The drawing under review shows one solid part. Ordinate dimensions are in mm from its lowest x, y, z. A direction names the side the tool comes from. Give positions to 0.01 mm unless a question says otherwise; leave off trailing zeros. Loops run counter-clockwise (first coordinate to the right, second up) from the corner with the lowest first, then second, coordinate; pieces in that order, holes last. Notation, with made-up numbers: (-4.75, -11.75) - (23.25, -11.75) arc R17 cw to (23.25, -7.75) - close; hole circle Ø8 at (16, -22). An arc over 180 degrees is marked (long way). Put each result on its own line as item: value. Start each with the question number.
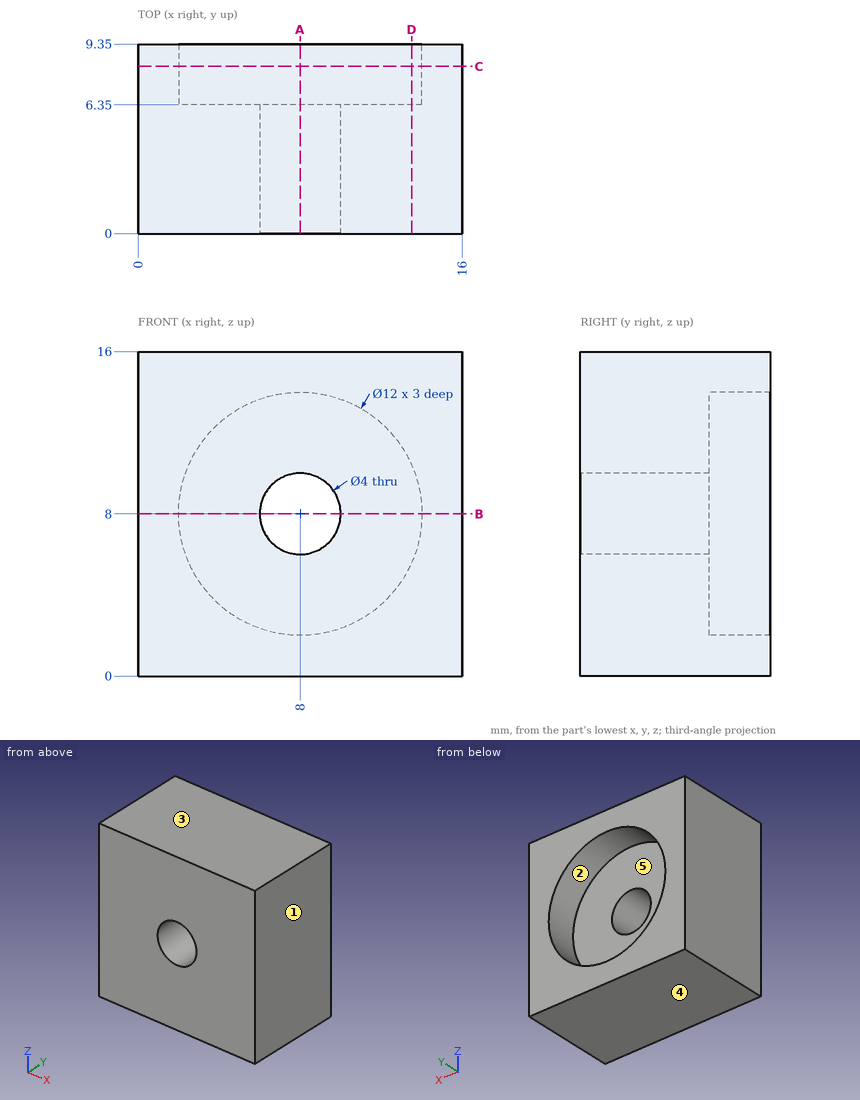
Item 1: Machinability: for the marked faces 4 and 5, which of the approach directions +Z, -Z, +X, -X, +Y, -Y give a long, thin tool a straight path to every point of the face, cutting with its end or side? Answer none if there is none.
Item 2: Consider section B-B (z = 8). State the section outline as (x, y) points, plus the area to 3 significant figures.
Item 3: For L1, parallel to Z at x = 8, y = 4.5; L2, parallel to Z at x = 8, y = 8.4, list the stretches that pass through material, from the lowest coordinate up. Write a range as from..to.
Item 4: Consider section C-C (y = 8.25). State the section outline as (x, z) points.
Item 5: Consider section D-D (x = 13.5). State the section outline as (y, z) points, plus the area to 3 significant figures.
Item 6: For P1, Ø4, axis at x = 13, y = 5.5, coming from the -Z side; P2, Ø2, axis at x = 4.5, z = 5, coming from the +Y side, all flat-tipped, find the tip position at first contact; note any pin that passes through.
Item 7: Consider section A-A (x = 8). State the section outline as (y, z) points, plus the area to 3 significant figures.
Item 8: Mouldability with a two-part tool opening along X and no side actions: class the marked faces 1, 2 and 3 as pulls with the +X half, pulls with the -X half, needs draft (parallel to the pull), parting line crosses it, or undercut.
Geometry says:
1. face 4: -Z, +X, -X, +Y, -Y
1. face 5: +Y
2. outline: (0, 0) - (6, 0) - (6, 6.35) - (2, 6.35) - (2, 9.35) - (0, 9.35) - close; (10, 0) - (16, 0) - (16, 9.35) - (14, 9.35) - (14, 6.35) - (10, 6.35) - close
2. area: 88.2 mm2
3. L1: z = 0..6, 10..16
3. L2: z = 0..2, 14..16
4. outline: (0, 0) - (16, 0) - (16, 16) - (0, 16) - close; hole circle Ø12 at (8, 8)
5. outline: (0, 0) - (9.35, 0) - (9.35, 5.6) - (6.35, 5.6) - (6.35, 10.4) - (9.35, 10.4) - (9.35, 16) - (0, 16) - close
5. area: 135 mm2
6. P1: stops at z = 0
6. P2: stops at y = 6.35
7. outline: (0, 0) - (9.35, 0) - (9.35, 2) - (6.35, 2) - (6.35, 6) - (0, 6) - close; (0, 10) - (6.35, 10) - (6.35, 14) - (9.35, 14) - (9.35, 16) - (0, 16) - close
7. area: 88.2 mm2
8. face 1: pulls with the +X half
8. face 2: undercut
8. face 3: needs draft
